The listing builds one solid part. Answer for the finished solid, in the listing's coordinates (mm). Face numbers are marked on the shaded views. A direction names the side the tool comes from. Give positions to 0.01 mm unless a question says otherwise; leave off trailing zeros. Write each loop counter-clockwise with the first axis right and the second up, starting at its lowest first coordinate (ties: lowest second). Pieces come first, ordered by that corner, then holes. Notation, with made-up numbers: (-11.75, 34.5) - (32.25, 34.5) arc R21 ccw to (32.25, 55.5) - close; hole circle Ø4 at (22.5, -15). An arc over 180 degrees is marked (long way). Answer in a Markdown table with one row per item. Add a question column.
Autodesk Inventor part; units mm, degrees
ref_plane "Work Plane1" through (0, 0, 24) normal (0, 0, 1) x (1, 0, 0)
ref_plane "YZ Plane" through (0, 0, 0) normal (1, 0, 0) x (0, 1, 0)
ref_plane "XZ Plane" through (0, 0, 0) normal (0, 1, 0) x (-1, 0, 0)
sketch "Sketch1" plane through (0, 0, 0) normal (0, 0, 1) x (1, 0, 0)
  line L0 (-6, -5) -> (6, -5)
  line L1 (6, -5) -> (6, 5)
  line L2 (6, 5) -> (-6, 5)
  line L3 (-6, 5) -> (-6, -5)
  line L4 (-6, -5) -> (6, 5) construction
  line L5 (6, -5) -> (-6, 5) construction
  circle A0 centre (0, -0.25) radius 2.125
  point P0 (0, 0)
  point P1 (0, 0)
  point P2 (0, 0)
  dimension "d0" = 12
  dimension "d1" = 10
  dimension "d2" = 4.25
  dimension "d18" = 0.25
extrude "Extrusion1" add sketch "Sketch1" along normal blind 30
sketch "Sketch2" plane through (-6, -5, 0) normal (0, -1, 0) x (1, 0, 0)
  circle A0 centre (6, 5) radius 2.1
  line L0 (0, 0) -> (12, 0)
  point P0 (6, 0)
  point P1 (6, 0)
  dimension "d5" = 4.2
  dimension "d6" = 5
sketch "Sketch3" plane through (0, 0, 0) normal (0, 0, -1) x (-1, 0, 0)
  line L0 (-6, -5) -> (-6, 5)
  line L1 (6, -5) -> (-6, -5)
  line L2 (6, 5) -> (6, -5)
  line L3 (-6, 5) -> (6, 5)
  circle A0 centre (0, -0.25) radius 2.125
  point P0 (0, 0)
extrude "Extrusion2" add sketch "Sketch3" against normal blind 10 contours A0
extrude "Extrusion3" cut sketch "Sketch2" against normal through all
ref_plane "Work Plane1" through (0, 0, 24) normal (0, 0, 1) x (1, 0, 0)
sketch "Sketch4" plane through (0, 0, 24) normal (0, 0, 1) x (1, 0, 0)
  line L0 (3.475, -2.0063) -> (0, -4.0126) construction
  line L1 (0, -4.0126) -> (-3.475, -2.0063) construction
  line L2 (-3.475, -2.0063) -> (-3.475, 2.0063)
  line L3 (-3.475, 2.0063) -> (0, 4.0126)
  line L4 (0, 4.0126) -> (3.475, 2.0063)
  line L5 (3.475, 2.0063) -> (3.475, -2.0063)
  line L6 (3.475, -2.0063) -> (3.475, -9.9564)
  line L7 (-3.475, -2.0063) -> (-3.475, -9.9564)
  line L8 (-3.475, -9.9564) -> (3.475, -9.9564)
  point P0 (0, 0)
  point P1 (0, 0)
  dimension "d12" = 6.95
extrude "Extrusion4" cut sketch "Sketch4" against normal blind 5
sketch "Sketch5" plane through (-6, -5, 0) normal (0, -1, 0) x (1, 0, 0)
  circle A0 centre (6, 5) radius 2.1
  circle A1 centre (6, 5) radius 3.625
  point P0 (6, 0)
  dimension "d15" = 7.25
extrude "Extrusion5" cut sketch "Sketch5" against normal blind 4
properties part number "mgn_screw_nut"
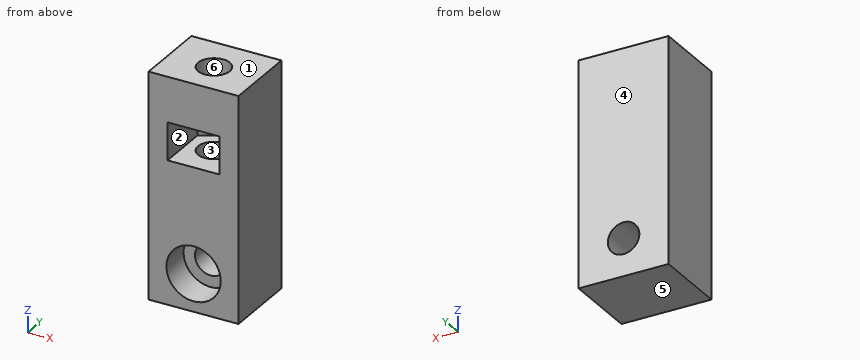
1. Given pin 1 Ø4.5 at (x, z) = (0, 5) entering from -Y; pin 2 Ø4 at (x, y) = (0, -0.25) entering from +Z, each flat-ended and moving along its own axis, determine where each tip first touches the part or whether it passes through.
2. Section A-A (z = 5) is taken. Give the vertices of the cut face in (x, y) (3 decimals), and give its area (3 significant figures).
3. The mould has two halves that part along Y. Classify the marked faces 4, 5 and 6: +Y half, -Y half, draft (parallel to the pull), parting line (faces both ways), or undercut.
4. Section C-C (y = -0.25) is taken. Give the vertices of the cut face in (x, z) (3 decimals), and give its area (3 significant figures).
5. Section D-D (y = -3.5) is taken. Give the vertices of the cut face in (x, z) (3 decimals).
6. Straight lines are drawn through the part: L1, parallel to Z at x = 0, y = -4.2 (3 decimals); L2, parallel to Z at x = 0, y = 3.45; L3, parallel to Y at x = 0, z = 14.75 (3 decimals). For each, find the intervals that lie inside material, in ascending order. Write a range as [from, to].
7. A tool of negligible diameter and unlimited length cuts with its end or side. For the marked faces 1, 2 and 3, from which of +Z, -Z, +X, -X, +Y, -Y can it reach the whole face along a straight path? Write none if from no direction.
8. Section B-B (x = -0.5) is taken. Give the vertices of the cut face in (y, z).
Geometry check:
| question | item | result |
|---|---|---|
| 1 | pin 1 | y = -1 |
| 1 | pin 2 | z = 10 |
| 2 | outline | (-6, -5) - (-3.625, -5) - (-3.625, -1) - (-2.1, -1) - (-2.1, 5) - (-6, 5) - close; (2.1, -1) - (3.625, -1) - (3.625, -5) - (6, -5) - (6, 5) - (2.1, 5) - close |
| 2 | area | 65.8 mm² |
| 3 | face 4 | +Y half |
| 3 | face 5 | draft |
| 3 | face 6 | undercut |
| 4 | outline | (-6, 0) - (6, 0) - (6, 30) - (2.125, 30) - (2.125, 24) - (3.475, 24) - (3.475, 19) - (2.125, 19) - (2.125, 10) - (-2.125, 10) - (-2.125, 19) - (-3.475, 19) - (-3.475, 24) - (-2.125, 24) - (-2.125, 30) - (-6, 30) - close; hole circle Ø4.2 at (0, 5) |
| 4 | area | 248 mm² |
| 5 | outline | (-6, 0) - (6, 0) - (6, 30) - (-6, 30) - close; hole circle Ø7.25 at (0, 5); hole (-3.475, 19) - (3.475, 19) - (3.475, 24) - (-3.475, 24) - close |
| 6 | L1 | [0, 1.375], [8.625, 19], [24, 30] |
| 6 | L2 | [0, 2.9], [7.1, 19], [24, 30] |
| 6 | L3 | [-5, -2.375], [1.875, 5] |
| 7 | face 1 | +Z, +X, -X, +Y, -Y |
| 7 | face 2 | -Y |
| 7 | face 3 | +Z |
| 8 | outline | (-5, 0) - (5, 0) - (5, 2.96) - (-1, 2.96) - (-1, 1.41) - (-5, 1.41) - close; (-5, 8.59) - (-1, 8.59) - (-1, 7.04) - (5, 7.04) - (5, 30) - (1.82, 30) - (1.82, 24) - (3.72, 24) - (3.72, 19) - (1.82, 19) - (1.82, 10) - (-2.32, 10) - (-2.32, 19) - (-5, 19) - close; (-5, 24) - (-2.32, 24) - (-2.32, 30) - (-5, 30) - close |
